Read the model definition and answer for the solid it produces. Units are mm, in the model's axes. A direction names the side the tool comes from. Coordinates: 2 decimals unless noted, no trailing zeros. Order: outer loops, then holes, each group sorted by start corner. A loop starts at its lowest first (then second) coordinate and runs counter-clockwise, first axis right, second up. Notation, with made-up numbers: M 51,56 L 110,56 A14 cw 110,78 Z; hole C 27.5,77 d10. An arc over 180 degrees is marked long. Use a Markdown table: item, result. Add a question column.
1) Find section C-C on y = 3.5. Write down the section's boundary in (x, z), plus the area to 3 significant figures.
2) The mould has two halves that part along Z. Classify faces 6 (the face through (21.8, -2.54, -4.43)), 7 (the face through (0.6, 5.48, 3.57)), 8 (the face through (-20.5, -3, -10)): released by +Z, released by -Z, zero draft, split by the parting line, or undercut.
3) Find section D-D on z = -11.5. Write down the section's boundary in (x, y).
4) Find the intervals of material crossed by probe 1 along Z at (x, y) = (-2.55, 18.5); probe 2 along X at (y, z) = (-3, -15); probe 3 along Z at (x, y) = (23, -3), in increasing order. Write a range as [from, to].
5) For faces 1 (the face through (-5, 5, 9)), 2 (the face through (14, 5, 3)), 3 (the face through (-23, 0, -11)), 4 (the face through (22.592, -2.535, -13.394)), 5 (the face through (24, -5, -11)), determine the directions among +Z, -Z, +X, -X, +Y, -Y from which every point of the face is accessible in a straight line to the end or side of a thin tool.
6) Each of these flat-tipped pins is pushed along its axis until it touches: pin 1 Ø3 at (x, y) = (21, 5) entering from +Z; pin 2 Ø12 at (x, y) = (-12, 8.5) entering from -Z; pin 3 Ø12 at (x, z) = (-7, -5.5) entering from +Y; pin 4 Ø1.5 at (y, z) = (13.5, 8.5) entering from +X. Where does it stop, or does it pass through?
7) Find section A-A on x = 23.9. Write down the section's boundary in (y, z), plus the area to 3 significant figures.
8) Find section B-B on z = -4.9. Write down the section's boundary in (x, y).
from build123d import *

# Parameters (mm, degrees)
SKETCH1_W           = 53
SKETCH1_H           = 32.5
BOSS_EXTRUDE1_DEPTH = 3
SKETCH2_W           = 6
SKETCH2_H           = 5
BOSS_EXTRUDE2_DEPTH = 21
FILLET1_R           = 1
SKETCH3_W           = 5
SKETCH3_H           = 32.5
BOSS_EXTRUDE3_DEPTH = 10
FILLET2_R           = 2
SKETCH4_R           = 2.15
CUT_EXTRUDE1_DEPTH  = 10
SKETCH5_R           = 1.5
CUT_EXTRUDE2_DEPTH  = 10


with BuildPart() as part:
    # Sketch1 → Boss-Extrude1 (new body)
    with BuildSketch(Plane.XY):
        with Locations((0, 5.25)):
            Rectangle(SKETCH1_W, SKETCH1_H)
    extrude(amount=BOSS_EXTRUDE1_DEPTH)

    # Sketch2 → Boss-Extrude2 (add)
    with BuildSketch(Plane(origin=(0, 0, 0), x_dir=(-1, 0, 0), z_dir=(0, 0, -1))):
        with Locations((23.5, -2.5)):
            Rectangle(SKETCH2_W, SKETCH2_H)
        with Locations((-23.5, -2.5)):
            Rectangle(SKETCH2_W, SKETCH2_H)
    extrude(amount=BOSS_EXTRUDE2_DEPTH)

    # Fillet1
    fillet1_edges = [part.edges().sort_by_distance(p)[0] for p in [
        (23.5, 0, 0),
        (23.5, -5, 0),
        (-23.5, 0, 0),
        (-23.5, -5, 0),
    ]]
    fillet(fillet1_edges, radius=FILLET1_R)

    # Sketch3 → Boss-Extrude3 (add)
    with BuildSketch(Plane.XY.offset(3)):
        with Locations((-2.5, 5.25)):
            Rectangle(SKETCH3_W, SKETCH3_H)
    extrude(amount=BOSS_EXTRUDE3_DEPTH)

    # Fillet2
    fillet2_edges = [part.edges().sort_by_distance(p)[0] for p in [
        (-5, 5.25, 3),
        (0, 5.25, 3),
    ]]
    fillet(fillet2_edges, radius=FILLET2_R)

    # Sketch4 → Cut-Extrude1 (cut)
    with BuildSketch(Plane.XZ.offset(5)):
        with Locations(Location((23.9, -4.9, 0), (0, 0, 270))):
            Circle(SKETCH4_R)
        with Locations(Location((23.9, -15.1, 0), (0, 0, 270))):
            Circle(SKETCH4_R)
        with Locations(Location((-23.9, -4.9, 0), (0, 0, 270))):
            Circle(SKETCH4_R)
        with Locations(Location((-23.9, -15.1, 0), (0, 0, 270))):
            Circle(SKETCH4_R)
    extrude(amount=-CUT_EXTRUDE1_DEPTH, mode=Mode.SUBTRACT)

    # Sketch5 → Cut-Extrude2 (cut)
    with BuildSketch(Plane(origin=(0, 0, 0), x_dir=(0, 0, -1), z_dir=(1, 0, 0))):
        with Locations(Location((-10, 18.5, 0), (0, 0, 90))):
            Circle(SKETCH5_R)
        with Locations(Location((-10, 3.5, 0), (0, 0, 90))):
            Circle(SKETCH5_R)
    extrude(amount=-CUT_EXTRUDE2_DEPTH, mode=Mode.SUBTRACT)


solid = part.part
Check result:
| question | item | result |
|---|---|---|
| 1 | outline | M -26.5,0 L 26.5,0 L 26.5,3 L 2,3 A2 cw 0,5 L 0,8.5 L -5,8.5 L -5,5 A2 cw -7,3 L -26.5,3 Z; M -5,11.5 L 0,11.5 L 0,13 L -5,13 Z |
| 1 | area | 196 mm2 |
| 2 | face 6 | undercut |
| 2 | face 7 | released by +Z |
| 2 | face 8 | zero draft |
| 3 | outline | M -26.5,-5 L -20.5,-5 L -20.5,0 L -26.5,0 Z; M 20.5,-5 L 26.5,-5 L 26.5,0 L 20.5,0 Z |
| 4 | probe 1 | z = [0, 8.5], [11.5, 13] |
| 4 | probe 2 | x = [-26.5, -26.05], [-21.75, -20.5], [20.5, 21.75], [26.05, 26.5] |
| 4 | probe 3 | z = [-21, -17.05], [-13.15, -6.85], [-2.95, 3] |
| 5 | face 1 | +Z, -X, +Y, -Y |
| 5 | face 2 | +Z, +X, +Y, -Y |
| 5 | face 3 | -Z, +X, -X, +Y |
| 5 | face 4 | +Y, -Y |
| 5 | face 5 | -Z, +X, -X, -Y |
| 6 | pin 1 | stops at z = 3 |
| 6 | pin 2 | stops at z = 0 |
| 6 | pin 3 | stops at y = 21.5 |
| 6 | pin 4 | stops at x = 0 |
| 7 | outline | M -11,0 L -6,0 A1 cw -5,-1 L -5,-2.75 L 0,-2.75 L 0,-1 A1 cw 1,0 L 21.5,0 L 21.5,3 L -11,3 Z; M -5,-21 L 0,-21 L 0,-17.25 L -5,-17.25 Z; M -5,-12.95 L 0,-12.95 L 0,-7.05 L -5,-7.05 Z |
| 7 | area | 160 mm2 |
| 8 | outline | M -26.5,-5 L -26.05,-5 L -26.05,0 L -26.5,0 Z; M -21.75,-5 L -20.5,-5 L -20.5,0 L -21.75,0 Z; M 20.5,-5 L 21.75,-5 L 21.75,0 L 20.5,0 Z; M 26.05,-5 L 26.5,-5 L 26.5,0 L 26.05,0 Z |
